Autodesk Fusion 360 part; units mm, degrees
sketch "Sketch1" plane through (0, 0, 0) normal (0, 0, 1) x (1, 0, 0)
  circle A0 centre (0, 0) radius 50
  circle A1 centre (0, 0) radius 47
  circle A2 centre (0, 0) radius 42
  dimension "d1" = 100
  dimension "d2" = -3
  dimension "d3" = -5
extrude "Extrude1" add sketch "Sketch1" along normal blind 5 contours A0 | A1 | A2
extrude "Extrude2" cut sketch "Sketch1" against normal blind 2 from surface at 5 contours A1
fillet "Fillet1" radius 1 4 edges at (-43.8194, 16.9959, 5) (-39.1577, -15.1878, 5) (-39.1577, -15.1878, 3) (-43.8194, 16.9959, 3)
CAD build for the part. Positions are in the model's coordinates, mm. Round coordinates to 2 decimals unless told otherwise and drop trailing zeros. Write each loop counter-clockwise with the first axis right and the second up, starting at its lowest first coordinate (ties: lowest second). Pieces come first, ordered by that corner, then holes. Notation, with made-up numbers: (-3.75, 23.5) - (45.25, 23.5) arc R30 cw to (45.25, 56.5) - close; hole circle Ø11 at (46, -31). An arc over 180 degrees is marked (long way). Write item = value, one per line. Start each with the question number.
Q1. Probe L1, parallel to Y at x = 0, z = 4; L2, parallel to Y at x = -34.5, z = 4.1; L3, parallel to X at y = 14.5, z = 3.8. List the from-to ranges inside material, lowest first. Write a range as from..to.
Q2. Band-saw the part on C-C (z = 1.4). Give the cut face in (x, y), then the cut area to 3 significant figures.
Q3. Mould opens along Y. For faces 1 (the flat face through (-19, 45, 5)), 2 (the cylindrical face through (47.69, -15.02, 2.46)), 3 (the flat face through (27, -34, 3)) say: pulls with the +Y half, pulls with the -Y half, needs draft (parallel to the pull), parting line crosses it, or undercut.
Q4. Drop flat-ended pins along their axis: pin 1 (3 mm diameter, centred on x = 13.5, y = 3.5, fed in from -Z); pin 2 (1.5 mm diameter, centred on y = 34, z = 4, fed in from -X). Give the stop position or say it passes through.
Answers below:
q1.L1 = -50..-47, -42..42, 47..50
q1.L2 = -36.19..-31.93, -23.94..23.94, 31.93..36.19
q1.L3 = -47.85..-44.69, -39.44..39.44, 44.69..47.85
q2.outline = circle Ø100 at (0, 0)
q2.area = 7,850 mm2
q3.face_1 = needs draft
q3.face_2 = parting line crosses it
q3.face_3 = undercut
q4.pin_1 = 0
q4.pin_2 = -37.34
